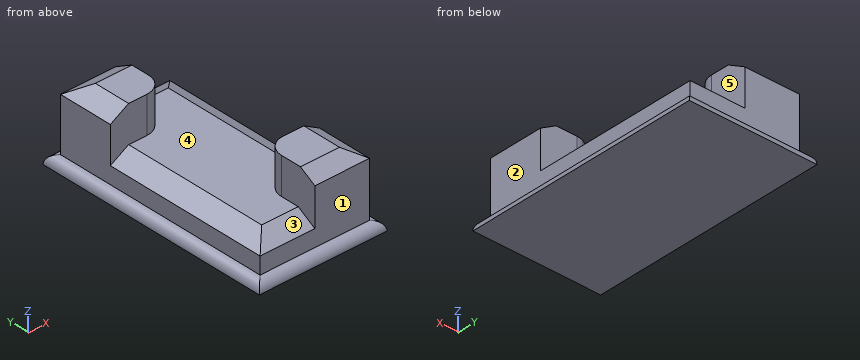
```python
from build123d import *

# Parameters (mm, degrees)
F1_DEPTH = 25.4
F0_W     = 88.9
F0_H     = 165.1
F2_DEPTH = 6.35
F3_DEPTH = 50.8
F4_R     = 6.34999
F5_SIZE2 = 7.3323484187
F5_SIZE  = 12.7
F6_SIZE2 = 7.3323484187
F6_SIZE  = 12.7
F7_SIZE2 = 10.9985226281
F7_SIZE  = 6.35


# Not quite as in the source:
# - a fillet or chamfer is up to 0.001 mm smaller than in the source, because OpenCascade refuses the exact size


with BuildPart() as f1:
    # F0 (on Top) → F1 (new body)
    with BuildSketch(Plane.XY):
        with BuildLine():
            Line((38.1, -38.1), (38.1, 76.2))
            Line((38.1, 76.2), (0, 76.2))
            Line((0, 76.2), (0, 50.8))
            ThreePointArc((0, 50.8), (-3.7197438789, 41.8197438789), (-12.7, 38.1))
            Line((-12.7, 38.1), (-38.1, 38.1))
            Line((-38.1, 38.1), (-38.1, -76.2))
            Line((-38.1, -76.2), (0.0100879326, -76.2))
            Line((0.0100879326, -76.2), (0.0100879326, -50.8))
            ThreePointArc((0.0100879326, -50.8), (3.7298318116, -41.8197438789), (12.7100879326, -38.1))
            Line((12.7100879326, -38.1), (38.1, -38.1))
        make_face()
    extrude(amount=F1_DEPTH)

    # F0 (on Top) → F2 (join)
    with BuildSketch(Plane.XY):
        Rectangle(F0_W, F0_H)
        Polygon((0, 76.2), (38.1, 76.2), (38.1, -38.1), (38.1, -76.2), (0.0100879326, -76.2), (-38.1, -76.2), (-38.1, 38.1), (-38.1, 76.2), align=None, mode=Mode.SUBTRACT)
    extrude(amount=F2_DEPTH)

    # F0 (on Top) → F3 (join)
    with BuildSketch(Plane.XY):
        with BuildLine():
            Line((0, 50.8), (0, 76.2))
            Line((0, 76.2), (-38.1, 76.2))
            Line((-38.1, 76.2), (-38.1, 38.1))
            Line((-38.1, 38.1), (-12.7, 38.1))
            ThreePointArc((-12.7, 38.1), (-3.7197438789, 41.8197438789), (0, 50.8))
        make_face()
        with BuildLine():
            Line((38.1, -76.2), (38.1, -38.1))
            Line((38.1, -38.1), (12.7100879326, -38.1))
            ThreePointArc((12.7100879326, -38.1), (3.7298318116, -41.8197438789), (0.0100879326, -50.8))
            Line((0.0100879326, -50.8), (0.0100879326, -76.2))
            Line((0.0100879326, -76.2), (38.1, -76.2))
        make_face()
    extrude(amount=F3_DEPTH)

    # F4 (radius 6.35 in the source; OpenCascade refuses exactly that, so slightly less here)
    f4_edges = [f1.edges().sort_by_distance(p)[0] for p in [
        (44.45, 0, 6.35),
        (0, 82.55, 6.35),
        (-44.45, 0, 6.35),
        (0, -82.55, 6.35),
    ]]
    fillet(f4_edges, radius=F4_R)

    # F5
    f5_edges = [f1.edges().sort_by_distance(p)[0] for p in [
        (-38.1, -19.05, 25.4),
        (-19.044956, -76.2, 25.4),
        (19.05, 76.2, 25.4),
        (38.1, 19.05, 25.4),
    ]]
    f5_side = f1.faces().sort_by_distance((4e-05, -0.002502, 25.4))[0]
    chamfer(f5_edges, length=F5_SIZE, length2=F5_SIZE2, reference=f5_side)

    # F6
    f6_edges = [f1.edges().sort_by_distance(p)[0] for p in [
        (-38.1, 57.15, 50.8),
        (-19.05, 76.2, 50.8),
    ]]
    f6_side = f1.faces().sort_by_distance((-19.446042, 57.546042, 50.8))[0]
    chamfer(f6_edges, length=F6_SIZE, length2=F6_SIZE2, reference=f6_side)

    # F7
    f7_edges = [f1.edges().sort_by_distance(p)[0] for p in [
        (38.1, -57.15, 50.8),
        (19.055044, -76.2, 50.8),
    ]]
    chamfer(f7_edges, length=F7_SIZE, length2=F7_SIZE2)


solid = f1.part
```
Work out the finished part from the listing and answer in its coordinate system (mm). Face numbers are marked on the shaded views. A direction names the side the tool comes from. Coordinates: 2 decimals unless noted, no trailing zeros. Write each loop counter-clockwise with the first axis right and the second up, starting at its lowest first coordinate (ties: lowest second). Pieces come first, ordered by that corner, then holes.
Q1. Each of these flat-tipped pins is pushed along its axis until it touches: pin 1 Ø10 at (y, z) = (-20, 24.5) entering from +X; pin 2 Ø12.5 at (y, z) = (-60.5, 31) entering from -X; pin 3 Ø19 at (x, z) = (7, 25) entering from -Y. Where does it stop, or does it pass through?
Q2. A cutting plane is placed at D-D, the plane z = 47. Give the vertices of the cut face in (x, y).
Q3. Find the intervals of material crossed by line 1 (Z direction, x = -8.5, y = -63); line 2 (X direction, y = 7.5, z = 6.5); line 3 (X direction, y = 65, z = 36), in increasing order.
Q4. Which of the six approach directions +Z, -Z, +X, -X, +Y, -Y give full straight-line access (tool end or side, diameter ignored) to the marked faces 1, 2, 3, 4 and 5?
Q5. A cutting plane is placed at A-A, the plane z = 33. Give the vertices of the cut face in (x, y).
Findings below:
1. pin 1: stops at x = 35.62
1. pin 2: stops at x = -26.53
1. pin 3: stops at y = -76.2
2. outline: (-31.98, 38.1) - (-12.7, 38.1) arc R12.7 ccw to (0, 50.8) - (0, 70.08) - (-31.98, 70.08) - close; (0.01, -71.78) - (33.68, -71.78) - (33.68, -38.1) - (12.71, -38.1) arc R12.7 ccw to (0.01, -50.8) - close
3. line 1: z = 0 to 25.4
3. line 2: x = -38.1 to 38.1
3. line 3: x = -38.1 to 0
4. face 1: +Z, +X, -X, -Y
4. face 2: +Z, +X, +Y, -Y
4. face 3: +Z, -X, -Y
4. face 4: +Z
4. face 5: +Z, +X, +Y
5. outline: (-38.1, 38.1) - (-12.7, 38.1) arc R12.7 ccw to (0, 50.8) - (0, 76.2) - (-38.1, 76.2) - close; (0.01, -76.2) - (38.1, -76.2) - (38.1, -38.1) - (12.71, -38.1) arc R12.7 ccw to (0.01, -50.8) - close
